Here's the drawing with two shaded views (mm, measured from the low corner). I have some questions. A direction names the side the tool comes from. Give positions to 0.01 mm unless a question says otherwise; leave off trailing zeros. Write each loop counter-clockwise with the first axis right and the second up, starting at its lowest first coordinate (ties: lowest second). Pieces come first, ordered by that corner, then holes. Notation, with made-up numbers: M 52.5,-11 L 83.5,-11 A17 ccw 83.5,-6 Z; hole C -33,45 d3. An arc over 180 degrees is marked long. Answer as a JSON object with one key per item and string values. Group by question number.
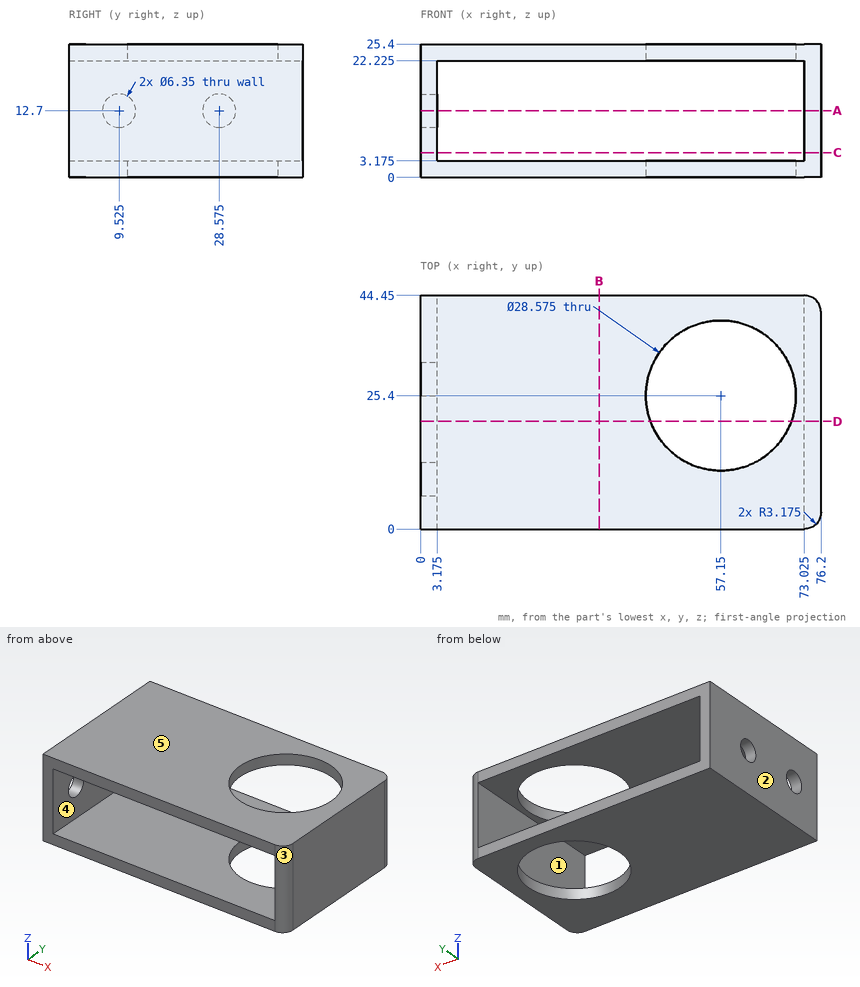
1) If we section it at B-B, the plane x = 34: List the corners of the cut face in (y, z) for me (3 decimals), plus the area to 3 significant figures.
2) For the marked faces 4 and 5, which set-ups out of +Z, -Z, +X, -X, +Y, -Y let a thin tool reach every point of the face, with its end or its side?
3) We'd pull the mould along X, two halves only. Please class the marked faces 1, 2 and 3: released by +X, released by -X, zero draft, split by the parting line, or undercut.
4) I'm going to push flat-ended pins straight in: pin 1 (5 mm diameter, centred on y = 9.525, z = 12.7, fed in from -X) (3 decimals); pin 2 (6 mm diameter, centred on x = 28, z = 6.5, fed in from -Y). Where does each tip first touch, or does it pass through?
5) If we section it at C-C, the plane z = 4.75: List the corners of the cut face in (x, y) for me (3 decimals), plus the area to 3 significant figures.
6) If we section it at D-D, the plane y = 20.5: List the corners of the cut face in (x, z) for me (3 decimals).
7) Please list where these lines run through material, in increasing order: line 1 along Y through (x, z) = (0.9, 12.7); line 2 along Z through (x, y) = (12.5, 42) (3 decimals); line 3 along X through (y, z) = (36, 5.5) (3 decimals). Write a range as from..to.
8) If we section it at A-A, the plane z = 12.7: List the corners of the cut face in (x, y) for me (3 decimals), plus the area to 3 significant figures.
Taken from the geometry:
{
 "1": {"outline": "M 0,0 L 44.45,0 L 44.45,3.175 L 0,3.175 Z; M 0,22.225 L 44.45,22.225 L 44.45,25.4 L 0,25.4 Z", "area": "282 mm²"},
 "2": {"face 4": "+Y, -Y", "face 5": "+Z, +X, -X, +Y, -Y"},
 "3": {"face 1": "undercut", "face 2": "released by -X", "face 3": "released by +X"},
 "4": {"pin 1": "x = 73.025", "pin 2": "through"},
 "5": {"outline": "M 0,0 L 3.175,0 L 3.175,44.45 L 0,44.45 Z; M 73.025,0 A3.175 ccw 76.2,3.175 L 76.2,41.275 A3.175 ccw 73.025,44.45 Z", "area": "278 mm²"},
 "6": {"outline": "M 0,0 L 43.729,0 L 43.729,3.175 L 3.175,3.175 L 3.175,22.225 L 43.729,22.225 L 43.729,25.4 L 0,25.4 Z; M 70.571,0 L 76.2,0 L 76.2,25.4 L 70.571,25.4 L 70.571,22.225 L 73.025,22.225 L 73.025,3.175 L 70.571,3.175 Z"},
 "7": {"line 1": "0..6.35, 12.7..25.4, 31.75..44.45", "line 2": "0..3.175, 22.225..25.4", "line 3": "0..3.175, 73.025..76.2"},
 "8": {"outline": "M 0,0 L 3.175,0 L 3.175,6.35 L 0,6.35 Z; M 0,12.7 L 3.175,12.7 L 3.175,25.4 L 0,25.4 Z; M 0,31.75 L 3.175,31.75 L 3.175,44.45 L 0,44.45 Z; M 73.025,0 A3.175 ccw 76.2,3.175 L 76.2,41.275 A3.175 ccw 73.025,44.45 Z", "area": "238 mm²"}
}
